from build123d import *

# Parameters (mm, degrees)
F0_R     = 4
F1_DEPTH = 20
F2_R     = 3.5
F3_DEPTH = 170
F4_R     = 1


with BuildPart() as f1:
    # F0 (on Right) → F1 (new body)
    with BuildSketch(Plane.YZ):
        Circle(F0_R)
    extrude(amount=F1_DEPTH)

    # F2 (on face) → F3 (join)
    with BuildSketch(Plane.YZ.offset(20)):
        Circle(F2_R)
    extrude(amount=F3_DEPTH)

    # F4
    f4_edges = [f1.edges().sort_by_distance(p)[0] for p in [
        (190, -3.5, 0),
    ]]
    fillet(f4_edges, radius=F4_R)


solid = f1.part
Input: part model. Units: mm. Frame: model coordinates. A direction names the side the tool comes from. Give positions to 0.01 mm unless a question says otherwise; leave off trailing zeros. Loops run counter-clockwise (first coordinate to the right, second up) from the corner with the lowest first, then second, coordinate; pieces in that order, holes last. Notation, with made-up numbers: (52.25, -32) - (87.25, -32) arc R25 cw to (87.25, -4) - close; hole circle Ø9 at (32, -39). An arc over 180 degrees is marked (long way). Use CSV: the item, a comma, the result in double quotes. Start each with the question number.
Item 1: Contact query for flat-ended pins moving along their axis: P1, Ø1.5, axis at x = 66, z = -2.5, coming from the +Y side; P2, Ø1.5, axis at x = 113, z = 2, coming from the -Y side; P3, Ø3, axis at x = 159, z = -0.5, coming from the -Y side. Output: stop coordinate, or through.
Item 2: Section A-A on z = 0. Return loops of the section in (x, y).
Item 3: Section C-C on x = 166.5. Return loops of the section in (y, z), then the cut area to 3 significant figures.
Item 4: Line query: line 1 (Y direction, x = 80.5, z = -0.5); line 2 (X direction, y = 1, z = 3.5); line 3 (Z direction, x = 99.5, y = 0.25). Output: solid intervals per line, ascending.
Item 5: Reachability of faces 1 (the cylindrical face through (103.317, 3.233, -1.341)), 2 (the cylindrical face through (9.86, -0.867, -3.905)) from +Z, -Z, +X, -X, +Y, -Y: full face, straight path, thin tool, end or side. Return the list, or none.
Ans:
1,P1,"stops at y = 3.03"
1,P2,"stops at y = -3.27"
1,P3,"stops at y = -3.5"
2,outline,"(0, -4) - (20, -4) - (20, -3.5) - (189, -3.5) arc R1 ccw to (190, -2.5) - (190, 2.5) arc R1 ccw to (189, 3.5) - (20, 3.5) - (20, 4) - (0, 4) - close"
3,outline,"circle Ø7 at (0, 0)"
3,area,"38.5 mm2"
4,line 1,"y = -3.46 to 3.46"
4,line 2,"x = 0 to 20"
4,line 3,"z = -3.49 to 3.49"
5,face 1,"+X"
5,face 2,"+X, -X"
